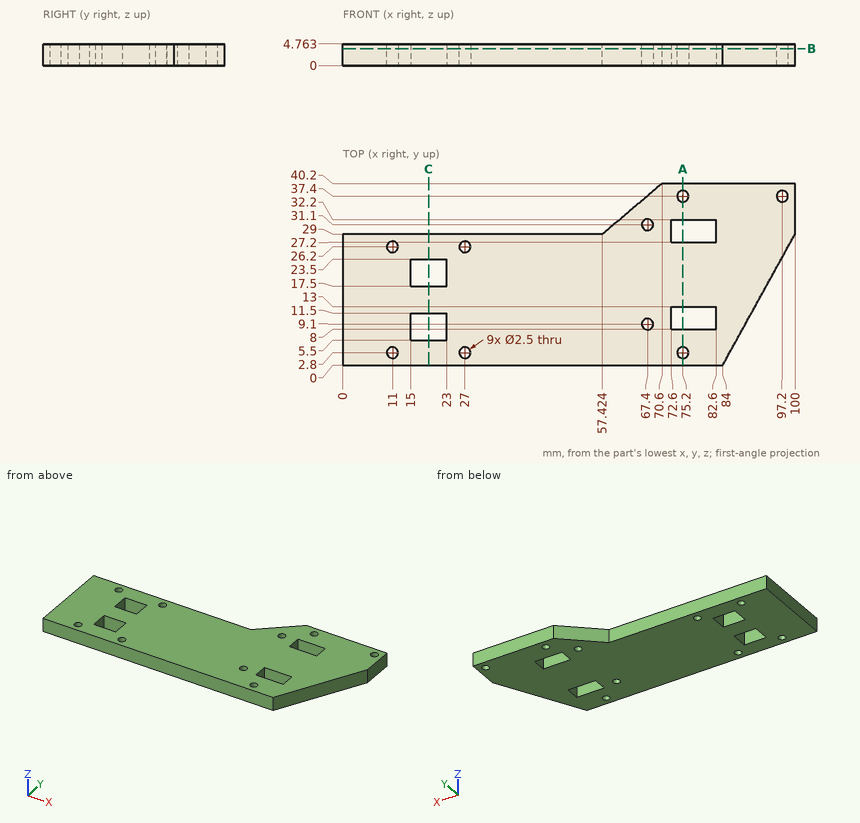
The drawing under review shows one solid part. Ordinate dimensions are in mm from its lowest x, y, z. Coordinates: 2 decimals unless noted, no trailing zeros. Loops run counter-clockwise (first coordinate to the right, second up) from the corner with the lowest first, then second, coordinate; pieces in that order, holes last. Notation, with made-up numbers: (13.5, 4) - (21.5, 4) arc R14 cw to (21.5, 13) - close; hole circle Ø3 at (55.5, -16). An arc over 180 degrees is marked (long way). Use CSV: the item, a comma, the result in double quotes. Start each with the question number.
1. Add section A-A on x = 75.2. Give the boundary of the cut face in (y, z), plus the area to 3 significant figures.
2. To check wall thickness, follow probe 1 along Y at (x, z) = (27, 1.75); probe 2 along Y at (x, z) = (75.2, 2.1); probe 3 along X at (y, z) = (3, 1.4) (1 decimal). State the ranges of each line that lie inside material, in increasing order.
3. Add section B-B on z = 3.75. Count the separate pieces of the cut face and the enclosed holes in it, plus the area to 3 significant figures.
4. Add section C-C on x = 19. Give the boundary of the cut face in (y, z).
5. Clearance check with flat-ended pins moving along their axes: pin 1 (1.4 mm diameter, centred on x = 19, z = 1.5, fed in from +Y); pin 2 (2.5 mm diameter, centred on y = 20, z = 2.5, fed in from +X) (1 decimal). State where each tip first meets the part, or that it passes through.
Resolved:
1,outline,"(0, 0) - (1.55, 0) - (1.55, 4.76) - (0, 4.76) - close; (4.05, 0) - (8, 0) - (8, 4.76) - (4.05, 4.76) - close; (13, 0) - (27.2, 0) - (27.2, 4.76) - (13, 4.76) - close; (32.2, 0) - (36.15, 0) - (36.15, 4.76) - (32.2, 4.76) - close; (38.65, 0) - (40.2, 0) - (40.2, 4.76) - (38.65, 4.76) - close"
1,area,"120 mm2"
2,probe 1,"0 to 1.55, 4.05 to 24.95, 27.45 to 29"
2,probe 2,"0 to 1.55, 4.05 to 8, 13 to 27.2, 32.2 to 36.15, 38.65 to 40.2"
2,probe 3,"0 to 9.8, 12.2 to 25.8, 28.2 to 74, 76.4 to 85.7"
3,separate pieces,"1"
3,enclosed holes,"13"
3,area,"2,830 mm2"
4,outline,"(0, 0) - (5.5, 0) - (5.5, 4.76) - (0, 4.76) - close; (11.5, 0) - (17.5, 0) - (17.5, 4.76) - (11.5, 4.76) - close; (23.5, 0) - (29, 0) - (29, 4.76) - (23.5, 4.76) - close"
5,pin 1,"y = 29"
5,pin 2,"x = 95.7"
